Part model, mm, in its own coordinate system. A direction names the side the tool comes from. Give positions to 0.01 mm unless a question says otherwise; leave off trailing zeros. Order: outer loops, then holes, each group sorted by start corner. A loop starts at its lowest first (then second) coordinate and runs counter-clockwise, first axis right, second up. Notation, with made-up numbers: (-15, 82.25) - (3, 82.25) arc R24 ccw to (3, 95.25) - close; hole circle Ø7 at (46, 73.5). An arc over 180 degrees is marked (long way). Use one line per item in the form item = value. Start each with the question number.
1. Pull direction Y, two halves, no side cores. Call faces 4 (the face through (0, 26, -3.937)), 5 (the face through (-9.426, 12.111, -1.709)), 6 (the face through (4.59, 37.27, -2.49)), 7 (the face through (-2, 35.688, -2)): +Y half, -Y half, draft (parallel to the pull), parting line (faces both ways), or undercut.
2. Band-saw the part on A-A, the plane x = 0. List the corners of the cut face in (y, z), plus the area to 3 significant figures.
3. Pin check, flat tips, straight feed: P1, Ø8, axis at x = -9.5, y = 16.5, coming from the +Z side; P2, Ø3, axis at x = -1, z = -2.5, coming from the -Y side; P3, Ø2, axis at x = 6.5, z = -2, coming from the +Y side; P4, Ø1, axis at y = 40.5, z = 1.5, coming from the +X side. Stop position of each tip, or through.
4. Drill centre lines: line 1 (Y direction, x = 3, z = -3.25); line 2 (Z direction, x = 0, y = 1.25); line 3 (Y direction, x = 9.5, z = -0.25). Where is each one in solid material? Low to high.
5. Band-saw the part on D-D, the plane z = -0.25. List the corners of the cut face in (x, y).
6. Band-saw the part on B-B, the plane z = -3.25. List the corners of the cut face in (x, y).
7. Tool access for faces 1 (the face through (4, 1, 6.878)), 2 (the face through (4, 2, 3)), 3 (the face through (-8.64, 37.34, -2.49)): list every direction of +Z, -Z, +X, -X, +Y, -Y with a clear straight run to the whole face (end or side of a thin tool).
8. Band-saw the part on C-C, the plane y = 23. List the corners of the cut face in (x, z), plus the area to 3 significant figures.
from build123d import *

# Parameters (mm, degrees)
SKETCH1_W                      = 30
SKETCH1_H                      = 10.814576134
BOSS_EXTRUDE1_DEPTH            = 2
SKETCH2_W                      = 30
SKETCH2_H                      = 2.938330184
BOSS_EXTRUDE2_DEPTH            = 50
CUT_EXTRUDE1_DEPTH             = 11.814576135
CUT_EXTRUDE2_REACH             = 4
SKETCH4_R                      = 1.6
CUT_EXTRUDE3_REACH             = 8.878
CUT_EXTRUDE3_DIRECTION_2_REACH = 5.937
FILLET1_R                      = 10


with BuildPart() as part:
    # Sketch1 → Boss-Extrude1 (new body)
    with BuildSketch(Plane(origin=(0, 0, 0), x_dir=(1, 0, 0), z_dir=(0, 1, 0))):
        with Locations((0, -1.470280193)):
            Rectangle(SKETCH1_W, SKETCH1_H)
    extrude(amount=BOSS_EXTRUDE1_DEPTH)

    # Sketch2 → Boss-Extrude2 (add)
    with BuildSketch(Plane(origin=(0, 2, 0), x_dir=(1, 0, 0), z_dir=(0, 1, 0))):
        with Locations((0, 2.467842782)):
            Rectangle(SKETCH2_W, SKETCH2_H)
    extrude(amount=BOSS_EXTRUDE2_DEPTH)

    # Sketch3 → Cut-Extrude1 (cut, through all)
    with BuildSketch(Plane(origin=(0, 0, -3.937007874), x_dir=(-1, 0, 0), z_dir=(0, 0, -1))):
        with BuildLine():
            Line((-2.975613291, 38.918099038), (7.024386709, 38.918099038))
            ThreePointArc((7.024386709, 38.918099038), (8.639544063, 37.302941685), (7.024386709, 35.687784331))
            Line((7.024386709, 35.687784331), (-2.975613291, 35.687784331))
            ThreePointArc((-2.975613291, 35.687784331), (-4.590770645, 37.302941685), (-2.975613291, 38.918099038))
        make_face()
        with BuildLine():
            Line((-2.975613291, 23.633431947), (7.024386709, 23.633431947))
            ThreePointArc((7.024386709, 23.633431947), (8.554876972, 22.102941685), (7.024386709, 20.572451422))
            Line((7.024386709, 20.572451422), (-2.975613291, 20.572451422))
            ThreePointArc((-2.975613291, 20.572451422), (-4.506103554, 22.102941685), (-2.975613291, 23.633431947))
        make_face()
    extrude(amount=-CUT_EXTRUDE1_DEPTH, mode=Mode.SUBTRACT)

    # Sketch4 → Cut-Extrude2 (cut, up to next)
    with BuildSketch(Plane(origin=(0, 2, 0), x_dir=(1, 0, 0), z_dir=(0, 1, 0)), mode=Mode.PRIVATE) as cut_extrude2_sk1:
        with Locations((10.61893739, -2.939445285)):
            Circle(SKETCH4_R)
    cut_extrude2_tool1 = extrude(cut_extrude2_sk1.sketch, amount=-CUT_EXTRUDE2_REACH, mode=Mode.PRIVATE) & part.part
    add(cut_extrude2_tool1.solids().sort_by_distance((10.618937, 2, 2.939445))[0], mode=Mode.SUBTRACT)
    # Sketch4 → Cut-Extrude2 (cut, up to next)
    with BuildSketch(Plane(origin=(0, 2, 0), x_dir=(1, 0, 0), z_dir=(0, 1, 0)), mode=Mode.PRIVATE) as cut_extrude2_sk2:
        with Locations((0, -2.939445285)):
            Circle(SKETCH4_R)
    cut_extrude2_tool2 = extrude(cut_extrude2_sk2.sketch, amount=-CUT_EXTRUDE2_REACH, mode=Mode.PRIVATE) & part.part
    add(cut_extrude2_tool2.solids().sort_by_distance((0, 2, 2.939445))[0], mode=Mode.SUBTRACT)

    # Sketch5 → Cut-Extrude3 (cut, up to next)
    with BuildSketch(Plane.XY, mode=Mode.PRIVATE) as cut_extrude3_sk1:
        Polygon((-4.080923029, -5.080850433), (-16.955695167, 36.332562893), (-18.585937562, -5.080850433), align=None)
    cut_extrude3_tool1 = extrude(cut_extrude3_sk1.sketch, amount=CUT_EXTRUDE3_REACH, mode=Mode.PRIVATE) & part.part
    add(cut_extrude3_tool1.solids().sort_by_distance((-13.207519, 8.723621, 0))[0], mode=Mode.SUBTRACT)

    # Sketch5 → Cut-Extrude3 direction 2 (cut, up to next)
    with BuildSketch(Plane.XY, mode=Mode.PRIVATE) as cut_extrude3_direction_2_sk1:
        Polygon((-4.080923029, -5.080850433), (-16.955695167, 36.332562893), (-18.585937562, -5.080850433), align=None)
    cut_extrude3_direction_2_tool1 = extrude(cut_extrude3_direction_2_sk1.sketch, amount=-CUT_EXTRUDE3_DIRECTION_2_REACH, mode=Mode.PRIVATE) & part.part
    add(cut_extrude3_direction_2_tool1.solids().sort_by_distance((-13.207519, 8.723621, 0))[0], mode=Mode.SUBTRACT)

    # Fillet1
    fillet1_edges = [part.edges().sort_by_distance(p)[0] for p in [
        (15, 52, -2.467842782),
        (-15, 52, -2.467842782),
        (-15, 30.041809827, -2.467842782),
    ]]
    fillet(fillet1_edges, radius=FILLET1_R)


solid = part.part
From the geometry:
q1.face_4 = draft
q1.face_5 = -Y half
q1.face_6 = undercut
q1.face_7 = undercut
q2.outline = (0, -3.94) - (20.57, -3.94) - (20.57, -1) - (2, -1) - (2, 1.34) - (0, 1.34) - close; (0, 4.54) - (2, 4.54) - (2, 6.88) - (0, 6.88) - close; (23.63, -3.94) - (35.69, -3.94) - (35.69, -1) - (23.63, -1) - close; (38.92, -3.94) - (52, -3.94) - (52, -1) - (38.92, -1) - close
q2.area = 144 mm²
q3.P1 = -1
q3.P2 = 0
q3.P3 = 51.99
q3.P4 = through
q4.line_1 = 0 to 20.57, 23.63 to 35.69, 38.92 to 52
q4.line_2 = -3.94 to 1.34, 4.54 to 6.88
q4.line_3 = 0 to 2
q5.outline = (-6.28, 2) - (-5.66, 0) - (15, 0) - (15, 2) - close
q6.outline = (-15, 31.56) arc R10 ccw to (-14.55, 28.59) - (-5.66, 0) - (15, 0) - (15, 42) arc R10 ccw to (5, 52) - (-5, 52) arc R10 ccw to (-15, 42) - close; hole (-7.02, 20.57) - (2.98, 20.57) arc R1.53 ccw to (2.98, 23.63) - (-7.02, 23.63) arc R1.53 ccw to start; hole (-7.02, 35.69) - (2.98, 35.69) arc R1.62 ccw to (2.98, 38.92) - (-7.02, 38.92) arc R1.62 ccw to start
q7.face_1 = +Z, +X, -X, +Y, -Y
q7.face_2 = +Z, +X, -X, +Y
q7.face_3 = +Z, -Z
q8.outline = (-12.81, -3.94) - (-8.26, -3.94) - (-8.26, -1) - (-12.81, -1) - close; (4.22, -3.94) - (15, -3.94) - (15, -1) - (4.22, -1) - close
q8.area = 45.0 mm²
